Input: part model. Units: mm. Frame: model coordinates. A direction names the side the tool comes from. Coordinates: 2 decimals unless noted, no trailing zeros. Order: outer loops, then holes, each group sorted by start corner. A loop starts at its lowest first (then second) coordinate and runs counter-clockwise, first axis right, second up. Notation, with made-up numbers: M -18.5,77 L 36.5,77 A28 ccw 36.5,114 Z; hole C -29.5,72 d11. An arc over 180 degrees is marked long. Answer in a Markdown table with one row per item.
from build123d import *

# Parameters (mm, degrees)
F0_W          = 44.45
F0_H          = 44.45
F1_DEPTH      = 12.7
F2_W          = 13.335
F2_H          = 5.08
F3_DEPTH      = 76.2
F4_R          = 3.175
F5_DEPTH      = 25.4
F6_T1_DEPTH   = 57.5141495789
F6_T3_DEPTH   = 57.5141495789
F7_T1_DEPTH   = 5.08
F7_T3_DEPTH   = 13.335
F7_T5_DEPTH   = 23.2241495789
F7_T11_DEPTH  = 19.8670747894
F7_T16_DEPTH  = 11.6120747894
F7_T24_DEPTH  = 19.8670747894
F7_T28_DEPTH  = 11.6120747894
F7_T36_DEPTH  = 11.6120747894
F7_T41_DEPTH  = 19.8670747894
F7_T49_DEPTH  = 11.6120747894
F7_T54_DEPTH  = 19.8670747894
F7_T61_DEPTH  = 19.8670747894
F7_T65_DEPTH  = 11.6120747894
F7_T73_DEPTH  = 11.6120747894
F7_T78_DEPTH  = 19.8670747894
F7_T85_DEPTH  = 19.8670747894
F7_T90_DEPTH  = 11.6120747894
F7_T98_DEPTH  = 11.6120747894
F7_T103_DEPTH = 19.8670747894
F8_R          = 3.175
F9_DEPTH      = 1.905


# Not quite as in the source:
# - a fillet or chamfer that OpenCascade refuses, or shapes differently, is made with other operations: its cross-section is extruded or revolved along the edge and cut away or added


with BuildPart() as f1:
    # F0 (on Top) → F1 (new body)
    with BuildSketch(Plane.XY):
        Rectangle(F0_W, F0_H)
    extrude(amount=F1_DEPTH)

    # F2 (on face) → F3 (cut)
    with BuildSketch(Plane.YZ.offset(22.225)):
        with Locations((0, 4.445)):
            Rectangle(F2_W, F2_H)
    extrude(amount=-F3_DEPTH, mode=Mode.SUBTRACT)

    # F4 (on face) → F5 (cut)
    with BuildSketch(Plane.XY.offset(12.7)):
        with Locations((10.795, 14.605)):
            Circle(F4_R)
        with Locations((-10.795, 14.605)):
            Circle(F4_R)
        with Locations((-10.795, -14.605)):
            Circle(F4_R)
        with Locations((10.795, -14.605)):
            Circle(F4_R)
        with Locations((-10.795, 0)):
            Circle(F4_R)
        with Locations((10.795, 0)):
            Circle(F4_R)
    extrude(amount=-F5_DEPTH, mode=Mode.SUBTRACT)

    # F6: chamfer of 2.54 on 10 edges, made by hand

    # F6_s2 → F6_t1 (cut)
    with BuildSketch(Plane.XZ.offset(-28.7570747894)):
        Polygon((22.225, 10.16), (19.685, 12.7), (22.225, 12.7), align=None)
        Polygon((-19.685, 12.7), (-22.225, 10.16), (-22.225, 12.7), align=None)
    extrude(amount=F6_T1_DEPTH, mode=Mode.SUBTRACT)

    # F6_s4 → F6_t3 (cut)
    with BuildSketch(Plane.YZ.offset(-28.7570747894)):
        Polygon((-22.225, 10.16), (-19.685, 12.7), (-22.225, 12.7), align=None)
        Polygon((19.685, 12.7), (22.225, 10.16), (22.225, 12.7), align=None)
    extrude(amount=F6_T3_DEPTH, mode=Mode.SUBTRACT)

    # F6_s5 → F6_t6 (revolve, cut)
    with BuildSketch(Plane.XZ.offset(14.605)):
        Polygon((-5.08, 12.7), (-7.62, 10.16), (-7.62, 12.7), align=None)
    revolve(axis=Axis((-10.795, -14.605, 12.7), (0, 0, 1)), mode=Mode.SUBTRACT)

    # F6_s7 → F6_t8 (revolve, cut)
    with BuildSketch(Plane.XZ):
        Polygon((-5.08, 12.7), (-7.62, 10.16), (-7.62, 12.7), align=None)
    revolve(axis=Axis((-10.795, 0, 12.7), (0, 0, 1)), mode=Mode.SUBTRACT)

    # F6_s9 → F6_t10 (revolve, cut)
    with BuildSketch(Plane.XZ.offset(14.605)):
        Polygon((16.51, 12.7), (13.97, 10.16), (13.97, 12.7), align=None)
    revolve(axis=Axis((10.795, -14.605, 12.7), (0, 0, 1)), mode=Mode.SUBTRACT)

    # F6_s11 → F6_t12 (revolve, cut)
    with BuildSketch(Plane.XZ):
        Polygon((16.51, 12.7), (13.97, 10.16), (13.97, 12.7), align=None)
    revolve(axis=Axis((10.795, 0, 12.7), (0, 0, 1)), mode=Mode.SUBTRACT)

    # F6_s13 → F6_t14 (revolve, cut)
    with BuildSketch(Plane.XZ.offset(-14.605)):
        Polygon((-5.08, 12.7), (-7.62, 10.16), (-7.62, 12.7), align=None)
    revolve(axis=Axis((-10.795, 14.605, 12.7), (0, 0, 1)), mode=Mode.SUBTRACT)

    # F6_s15 → F6_t16 (revolve, cut)
    with BuildSketch(Plane.XZ.offset(-14.605)):
        Polygon((16.51, 12.7), (13.97, 10.16), (13.97, 12.7), align=None)
    revolve(axis=Axis((10.795, 14.605, 12.7), (0, 0, 1)), mode=Mode.SUBTRACT)

    # F7: chamfer of 2.54 on 12 edges, made by hand

    # F7_s2 → F7_t1 (cut)
    with BuildSketch(Plane.XY.offset(1.905)):
        Polygon((22.225, 9.2075), (19.685, 6.6675), (22.225, 6.6675), align=None)
        Polygon((22.225, -9.2075), (19.685, -6.6675), (22.225, -6.6675), align=None)
        Polygon((-19.685, 6.6675), (-22.225, 9.2075), (-22.225, 6.6675), align=None)
        Polygon((-19.685, -6.6675), (-22.225, -9.2075), (-22.225, -6.6675), align=None)
    extrude(amount=F7_T1_DEPTH, mode=Mode.SUBTRACT)

    # F7_s4 → F7_t3 (cut)
    with BuildSketch(Plane.XZ.offset(-6.6675)):
        Polygon((22.225, -0.635), (19.685, 1.905), (22.225, 1.905), align=None)
        Polygon((22.225, 9.525), (19.685, 6.985), (22.225, 6.985), align=None)
        Polygon((-19.685, 6.985), (-22.225, 9.525), (-22.225, 6.985), align=None)
        Polygon((-19.685, 1.905), (-22.225, -0.635), (-22.225, 1.905), align=None)
    extrude(amount=F7_T3_DEPTH, mode=Mode.SUBTRACT)

    # F7_s6 → F7_t5 (cut)
    with BuildSketch(Plane.XY.offset(-6.5320747894)):
        Polygon((-19.685, -22.225), (-22.225, -19.685), (-22.225, -22.225), align=None)
        Polygon((22.225, -19.685), (19.685, -22.225), (22.225, -22.225), align=None)
        Polygon((22.225, 19.685), (19.685, 22.225), (22.225, 22.225), align=None)
        Polygon((-19.685, 22.225), (-22.225, 19.685), (-22.225, 22.225), align=None)
    extrude(amount=F7_T5_DEPTH, mode=Mode.SUBTRACT)


with BuildPart() as f7_tool9:
    # F7_s10 → F7_t11 (new body)
    with BuildSketch(Plane.XZ.offset(6.6675)):
        Polygon((22.225, -0.635), (19.685, 1.905), (22.225, 1.905), align=None)
    extrude(amount=-F7_T11_DEPTH)

    split(bisect_by=Plane.XY, keep=Keep.TOP)

    split(bisect_by=Plane.XZ.offset(-6.6675), keep=Keep.BOTTOM)


with BuildPart() as f7_tool14:
    # F7_s15 → F7_t16 (new body)
    with BuildSketch(Plane.XY.offset(-4.6270747894)):
        Polygon((22.225, 9.2075), (19.685, 6.6675), (22.225, 6.6675), align=None)
    extrude(amount=F7_T16_DEPTH)

    split(bisect_by=Plane.XY, keep=Keep.TOP)

    split(bisect_by=Plane.XY.offset(1.905), keep=Keep.BOTTOM)


with BuildPart() as f7_tool9_1:
    add(f7_tool9.part)

    # F7_t19: intersect F7_tool14
    add(f7_tool14.part, mode=Mode.INTERSECT)


with BuildPart() as f1_1:
    add(f1.part)

    # F7_t7: cut F7_tool9
    add(f7_tool9_1.part, mode=Mode.SUBTRACT)


with BuildPart() as f7_tool22:
    # F7_s23 → F7_t24 (new body)
    with BuildSketch(Plane.XZ.offset(-13.1995747894)):
        Polygon((22.225, 9.525), (19.685, 6.985), (22.225, 6.985), align=None)
    extrude(amount=F7_T24_DEPTH)

    split(bisect_by=Plane.XZ.offset(-6.6675), keep=Keep.BOTTOM)


with BuildPart() as f7_tool26:
    # F7_s27 → F7_t28 (new body)
    with BuildSketch(Plane.XY.offset(1.905)):
        Polygon((22.225, 9.2075), (19.685, 6.6675), (22.225, 6.6675), align=None)
    extrude(amount=F7_T28_DEPTH)

    split(bisect_by=Plane(origin=(16.1925, 0, 16.1925), x_dir=(0, 1, 0), z_dir=(-0.7071067812, 0, -0.7071067812)), keep=Keep.TOP)

    split(bisect_by=Plane.XY.offset(6.985), keep=Keep.TOP)


with BuildPart() as f7_tool22_1:
    add(f7_tool22.part)

    # F7_t31: intersect F7_tool26
    add(f7_tool26.part, mode=Mode.INTERSECT)


with BuildPart() as f1_2:
    add(f1_1.part)

    # F7_t20: cut F7_tool22
    add(f7_tool22_1.part, mode=Mode.SUBTRACT)


with BuildPart() as f7_tool34:
    # F7_s35 → F7_t36 (new body)
    with BuildSketch(Plane.XY.offset(6.985)):
        Polygon((22.225, -9.2075), (19.685, -6.6675), (22.225, -6.6675), align=None)
    extrude(amount=-F7_T36_DEPTH)

    split(bisect_by=Plane.XY, keep=Keep.TOP)

    split(bisect_by=Plane.XY.offset(1.905), keep=Keep.BOTTOM)


with BuildPart() as f7_tool39:
    # F7_s40 → F7_t41 (new body)
    with BuildSketch(Plane.XZ.offset(13.1995747894)):
        Polygon((22.225, -0.635), (19.685, 1.905), (22.225, 1.905), align=None)
    extrude(amount=-F7_T41_DEPTH)

    split(bisect_by=Plane.XY, keep=Keep.TOP)

    split(bisect_by=Plane.XZ.offset(6.6675), keep=Keep.TOP)


with BuildPart() as f7_tool34_1:
    add(f7_tool34.part)

    # F7_t44: intersect F7_tool39
    add(f7_tool39.part, mode=Mode.INTERSECT)


with BuildPart() as f1_3:
    add(f1_2.part)

    # F7_t32: cut F7_tool34
    add(f7_tool34_1.part, mode=Mode.SUBTRACT)


with BuildPart() as f7_tool47:
    # F7_s48 → F7_t49 (new body)
    with BuildSketch(Plane.XY.offset(13.5170747894)):
        Polygon((22.225, -9.2075), (19.685, -6.6675), (22.225, -6.6675), align=None)
    extrude(amount=-F7_T49_DEPTH)

    split(bisect_by=Plane(origin=(16.1925, 0, 16.1925), x_dir=(0, 1, 0), z_dir=(-0.7071067812, 0, -0.7071067812)), keep=Keep.TOP)

    split(bisect_by=Plane.XY.offset(6.985), keep=Keep.TOP)


with BuildPart() as f7_tool52:
    # F7_s53 → F7_t54 (new body)
    with BuildSketch(Plane.XZ.offset(-6.6675)):
        Polygon((22.225, 9.525), (19.685, 6.985), (22.225, 6.985), align=None)
    extrude(amount=F7_T54_DEPTH)

    split(bisect_by=Plane.XZ.offset(6.6675), keep=Keep.TOP)


with BuildPart() as f7_tool47_1:
    add(f7_tool47.part)

    # F7_t56: intersect F7_tool52
    add(f7_tool52.part, mode=Mode.INTERSECT)


with BuildPart() as f1_4:
    add(f1_3.part)

    # F7_t45: cut F7_tool47
    add(f7_tool47_1.part, mode=Mode.SUBTRACT)


with BuildPart() as f7_tool59:
    # F7_s60 → F7_t61 (new body)
    with BuildSketch(Plane.XZ.offset(-13.1995747894)):
        Polygon((-19.685, 6.985), (-22.225, 9.525), (-22.225, 6.985), align=None)
    extrude(amount=F7_T61_DEPTH)

    split(bisect_by=Plane.XZ.offset(-6.6675), keep=Keep.BOTTOM)


with BuildPart() as f7_tool63:
    # F7_s64 → F7_t65 (new body)
    with BuildSketch(Plane.XY.offset(1.905)):
        Polygon((-19.685, 6.6675), (-22.225, 9.2075), (-22.225, 6.6675), align=None)
    extrude(amount=F7_T65_DEPTH)

    split(bisect_by=Plane.XY.offset(6.985), keep=Keep.TOP)

    split(bisect_by=Plane(origin=(-16.1925, 0, 16.1925), x_dir=(0, 1, 0), z_dir=(0.7071067812, 0, -0.7071067812)), keep=Keep.TOP)


with BuildPart() as f7_tool59_1:
    add(f7_tool59.part)

    # F7_t68: intersect F7_tool63
    add(f7_tool63.part, mode=Mode.INTERSECT)


with BuildPart() as f1_5:
    add(f1_4.part)

    # F7_t57: cut F7_tool59
    add(f7_tool59_1.part, mode=Mode.SUBTRACT)


with BuildPart() as f7_tool71:
    # F7_s72 → F7_t73 (new body)
    with BuildSketch(Plane.XY.offset(13.5170747894)):
        Polygon((-19.685, -6.6675), (-22.225, -9.2075), (-22.225, -6.6675), align=None)
    extrude(amount=-F7_T73_DEPTH)

    split(bisect_by=Plane.XY.offset(6.985), keep=Keep.TOP)

    split(bisect_by=Plane(origin=(-16.1925, 0, 16.1925), x_dir=(0, 1, 0), z_dir=(0.7071067812, 0, -0.7071067812)), keep=Keep.TOP)


with BuildPart() as f7_tool76:
    # F7_s77 → F7_t78 (new body)
    with BuildSketch(Plane.XZ.offset(-6.6675)):
        Polygon((-19.685, 6.985), (-22.225, 9.525), (-22.225, 6.985), align=None)
    extrude(amount=F7_T78_DEPTH)

    split(bisect_by=Plane.XZ.offset(6.6675), keep=Keep.TOP)


with BuildPart() as f7_tool71_1:
    add(f7_tool71.part)

    # F7_t80: intersect F7_tool76
    add(f7_tool76.part, mode=Mode.INTERSECT)


with BuildPart() as f1_6:
    add(f1_5.part)

    # F7_t69: cut F7_tool71
    add(f7_tool71_1.part, mode=Mode.SUBTRACT)


with BuildPart() as f7_tool83:
    # F7_s84 → F7_t85 (new body)
    with BuildSketch(Plane.XZ.offset(6.6675)):
        Polygon((-19.685, 1.905), (-22.225, -0.635), (-22.225, 1.905), align=None)
    extrude(amount=-F7_T85_DEPTH)

    split(bisect_by=Plane.XY, keep=Keep.TOP)

    split(bisect_by=Plane.XZ.offset(-6.6675), keep=Keep.BOTTOM)


with BuildPart() as f7_tool88:
    # F7_s89 → F7_t90 (new body)
    with BuildSketch(Plane.XY.offset(-4.6270747894)):
        Polygon((-19.685, 6.6675), (-22.225, 9.2075), (-22.225, 6.6675), align=None)
    extrude(amount=F7_T90_DEPTH)

    split(bisect_by=Plane.XY, keep=Keep.TOP)

    split(bisect_by=Plane.XY.offset(1.905), keep=Keep.BOTTOM)


with BuildPart() as f7_tool83_1:
    add(f7_tool83.part)

    # F7_t93: intersect F7_tool88
    add(f7_tool88.part, mode=Mode.INTERSECT)


with BuildPart() as f1_7:
    add(f1_6.part)

    # F7_t81: cut F7_tool83
    add(f7_tool83_1.part, mode=Mode.SUBTRACT)


with BuildPart() as f7_tool96:
    # F7_s97 → F7_t98 (new body)
    with BuildSketch(Plane.XY.offset(6.985)):
        Polygon((-19.685, -6.6675), (-22.225, -9.2075), (-22.225, -6.6675), align=None)
    extrude(amount=-F7_T98_DEPTH)

    split(bisect_by=Plane.XY, keep=Keep.TOP)

    split(bisect_by=Plane.XY.offset(1.905), keep=Keep.BOTTOM)


with BuildPart() as f7_tool101:
    # F7_s102 → F7_t103 (new body)
    with BuildSketch(Plane.XZ.offset(13.1995747894)):
        Polygon((-19.685, 1.905), (-22.225, -0.635), (-22.225, 1.905), align=None)
    extrude(amount=-F7_T103_DEPTH)

    split(bisect_by=Plane.XY, keep=Keep.TOP)

    split(bisect_by=Plane.XZ.offset(6.6675), keep=Keep.TOP)


with BuildPart() as f7_tool96_1:
    add(f7_tool96.part)

    # F7_t106: intersect F7_tool101
    add(f7_tool101.part, mode=Mode.INTERSECT)


with BuildPart() as f1_8:
    add(f1_7.part)

    # F7_t94: cut F7_tool96
    add(f7_tool96_1.part, mode=Mode.SUBTRACT)

    # F8 (on face) → F9 (join, through all)
    with BuildSketch(Plane(origin=(0, 0, 0), x_dir=(1, 0, 0), z_dir=(0, 0, -1))):
        with Locations((10.795, 0)):
            Circle(F8_R)
        with Locations((-10.795, 0)):
            Circle(F8_R)
    extrude(amount=-F9_DEPTH)


solid = f1_8.part
1) Contact query for flat-ended pins moving along their axis: pin 1 (7.5 mm diameter, centred on x = -10.795, y = 0, fed in from +Z) (3 decimals); pin 2 (4 mm diameter, centred on x = -10.795, y = -14.605, fed in from -Z). Output: stop coordinate, or through.
Resolved:
| item | result |
|---|---|
| pin 1 | stops at z = 10.735 |
| pin 2 | passes through |
2) Reachability of faces 1 (the face through (20.973, 7.955, 4.696)), 2 (the face through (0, 6.668, 4)), 3 (the face through (-20.94, -7.92, 4.83)), 4 (the face through (12.26, 11.79, 5.15)) from +Z, -Z, +X, -X, +Y, -Y: full face, straight path, thin tool, end or side. Return the list, or none.
Resolved:
| item | result |
|---|---|
| face 1 | +X |
| face 2 | +X, -X |
| face 3 | -X |
| face 4 | +Z, -Z |
3) Cut plane C-C, the plane z = 7.5. State how many separate pieces and enclosed holes the cut face has, and give its area (3 significant figures).
Resolved:
| item | result |
|---|---|
| separate pieces | 1 |
| enclosed holes | 6 |
| area | 1,710 mm2 |
4) Cut plane B-B, the plane x = 18.5. Output: boundary loops of the cut face in (y, z) (1 decimal), and give its area (3 significant figures).
Resolved:
| item | result |
|---|---|
| outline | M -22.2,0 L 22.2,0 L 22.2,10.2 L 19.7,12.7 L -19.7,12.7 L -22.2,10.2 Z; hole M -6.7,1.9 L 6.7,1.9 L 6.7,7 L -6.7,7 Z |
| area | 490 mm2 |
5) Material intervals for probe 1 along Y at (x, z) = (6.5, 3.75) (1 decimal); probe 2 along Z at (x, y) = (18, 6) (3 decimals); probe 3 along Y at (x, z) = (-10.5, 11.25) (3 decimals), sorted ascending.
Resolved:
| item | result |
|---|---|
| probe 1 | y = -22.2 to -6.7, 6.7 to 22.2 |
| probe 2 | z = 0 to 1.905, 6.985 to 12.7 |
| probe 3 | y = -21.135 to -18.86, -10.35 to -4.255, 4.255 to 10.35, 18.86 to 21.135 |
6) Mould query, pull axis Z, two halves, no side actions, for faces 5 (the face through (-13.31, 12.67, 5.15)), 6 (the face through (8.178, -2.007, 10.283)), 7 (the face through (-20.94, 7.92, 4.7)). Classes: +Z half, -Z half, draft (parallel to the pull), parting line (faces both ways), or undercut.
Resolved:
| item | result |
|---|---|
| face 5 | draft |
| face 6 | +Z half |
| face 7 | undercut |
7) Cut plane A-A, the plane y = 0. Output: boundary loops of the cut face in (x, z) (3 decimals).
Resolved:
| item | result |
|---|---|
| outline | M -22.225,9.525 L -19.685,6.985 L -13.97,6.985 L -13.97,10.16 L -16.51,12.7 L -19.685,12.7 L -22.225,10.16 Z; M -21.59,0 L 21.59,0 L 19.685,1.905 L -19.685,1.905 Z; M -7.62,6.985 L 7.62,6.985 L 7.62,10.16 L 5.08,12.7 L -5.08,12.7 L -7.62,10.16 Z; M 13.97,6.985 L 19.685,6.985 L 22.225,9.525 L 22.225,10.16 L 19.685,12.7 L 16.51,12.7 L 13.97,10.16 Z |
